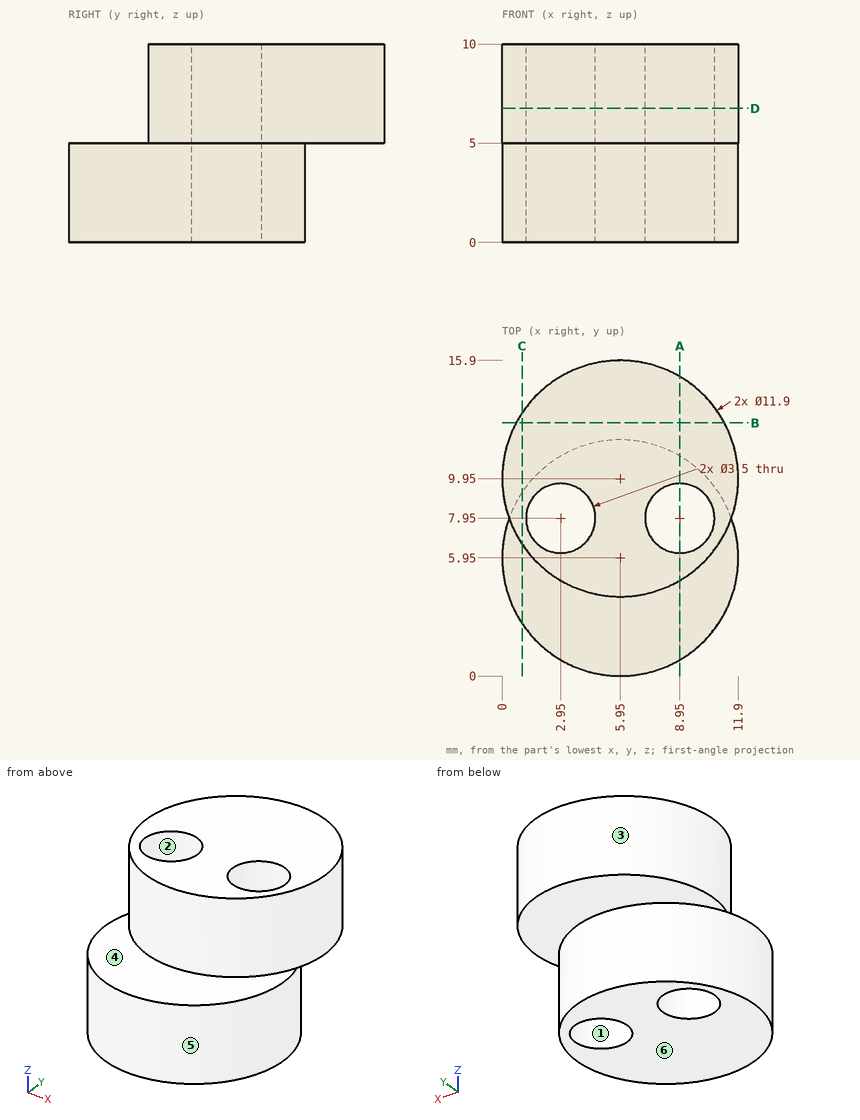
The figure shows three views and two pictorial views of one solid part (mm, origin at its lowest corner). Answer the questions. A direction names the side the tool comes from. Round coordinates to 2 decimals unless told otherwise and drop trailing zeros. Loops run counter-clockwise (first coordinate to the right, second up) from the corner with the lowest first, then second, coordinate; pieces in that order, holes last. Notation, with made-up numbers: M 63,35.25 L 70,35.25 A27 cw 70,54.25 Z; hole C -8.5,41 d7. An arc over 180 degrees is marked long. Write each question's results on one line, items separated by ' | '. Start each with the question number.
1) Which of the six approach directions +Z, -Z, +X, -X, +Y, -Y give full straight-line access (tool end or side, diameter ignored) to the marked faces 5 and 6?
2) Straight lines are drawn through the part: probe 1 along X at (y, z) = (7.95, 7.75); probe 2 along X at (y, z) = (7, 2.75); probe 3 along Z at (x, y) = (3.5, 2.75). For each, find the intervals that lie inside material, in ascending order.
3) Find section B-B on y = 12.75. Write down the section's boundary in (x, z), plus the area to 3 significant figures.
4) Determine the mould class of the marked faces 1, 2, 3 and 4 for opening direction X: pulls with the +X half, pulls with the -X half, needs draft (parallel to the pull), parting line crosses it, or undercut.
5) Find section A-A on x = 8.95. Write down the section's boundary in (y, z), plus the area to 3 significant figures.
6) Find section D-D on z = 6.75. Write down the section's boundary in (x, y), plus the area to 3 significant figures.
7) Find section C-C on x = 1. Write down the section's boundary in (y, z), plus the area to 3 significant figures.
8) Each of these flat-tipped pins is pushed along its axis until it touches: pin 1 (1.5 mm diameter, centred on x = 3.5, z = 2, fed in from -Y); pin 2 (1 mm diameter, centred on x = 1.5, y = 13, fed in from -Z); pin 3 (1.5 mm diameter, centred on x = 8, z = 1.5, fed in from +Y). Where does it stop, or does it pass through?
Final values:
1) face 5: -Z | face 6: -Z, +X, -X, +Y, -Y
2) probe 1: 0.35 to 1.2, 4.7 to 7.2, 10.7 to 11.55 | probe 2: 0.09 to 1.48, 4.42 to 7.48, 10.42 to 11.81 | probe 3: 0 to 5
3) outline: M 0.7,5 L 11.2,5 L 11.2,10 L 0.7,10 Z | area: 52.5 mm²
4) face 1: undercut | face 2: undercut | face 3: parting line crosses it | face 4: needs draft
5) outline: M 0.81,0 L 6.2,0 L 6.2,10 L 4.81,10 L 4.81,5 L 0.81,5 Z; M 9.7,0 L 11.09,0 L 11.09,5 L 15.09,5 L 15.09,10 L 9.7,10 Z | area: 67.8 mm²
6) outline: C 5.95,9.95 d11.9; hole C 2.95,7.95 d3.5; hole C 8.95,7.95 d3.5 | area: 92.0 mm²
7) outline: M 2.65,0 L 9.25,0 L 9.25,5 L 13.25,5 L 13.25,10 L 6.65,10 L 6.65,5 L 2.65,5 Z | area: 66.0 mm²
8) pin 1: y = 0.25 | pin 2: z = 5 | pin 3: y = 11.76
